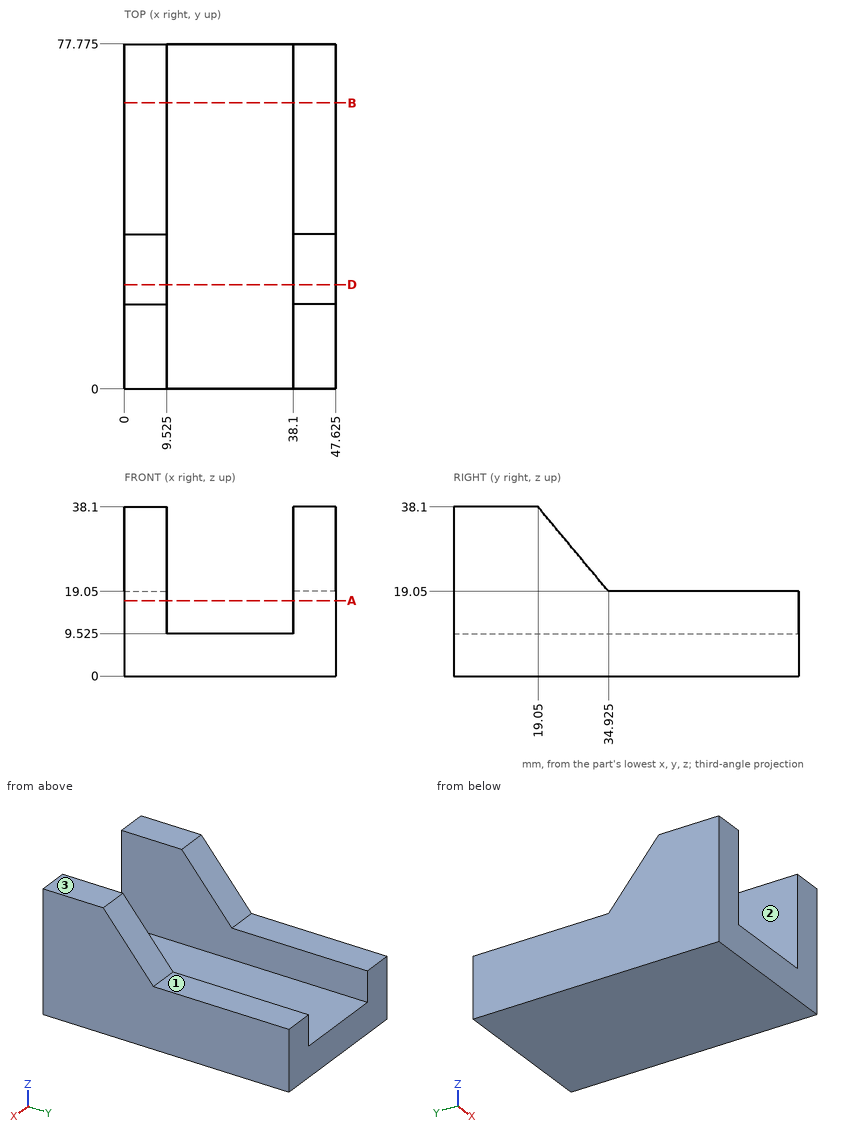
Geometry check sheet. Reference: drawing and pictorial views, mm from the part's lowest x, y, z. A direction names the side the tool comes from. Round coordinates to 2 decimals unless told otherwise and drop trailing zeros. Order: outer loops, then holes, each group sorted by start corner. A loop starts at its lowest first (then second) coordinate and runs counter-clockwise, first axis right, second up.
Q1. Depth check by flat-ended pin: P1, Ø10.5, axis at x = 44.5, y = 51, coming from the +Z side; P2, Ø8.5, axis at x = 18, y = 49, coming from the +Z side (3 decimals). Enter the tip coordinate at first touch or a pass-through.
Filled sheet:
P1: stops at z = 19.05
P2: stops at z = 9.525
Q2. Set-up check for the marked faces 1, 2 and 3: record each of +Z, -Z, +X, -X, +Y, -Y from which the full face is reachable in a straight line by a thin tool's end or side.
Filled sheet:
face 1: +Z, +X, -X, +Y
face 2: +Z, +Y, -Y
face 3: +Z, +X, -X, +Y, -Y
Q3. Cross-section at A-A, the plane z = 17. Enter the section's corners in (x, y) (1 decimal).
Filled sheet:
outline: (0, 0) - (9.5, 0) - (9.5, 77.8) - (0, 77.8) - close; (38.1, 0) - (47.6, 0) - (47.6, 77.8) - (38.1, 77.8) - close
Q4. Cross-section at B-B, the plane y = 64.5. Enter the section's corners in (x, z) (3 decimals).
Filled sheet:
outline: (0, 0) - (47.625, 0) - (47.625, 19.05) - (38.1, 19.05) - (38.1, 9.525) - (9.525, 9.525) - (9.525, 19.05) - (0, 19.05) - close
Q5. Cross-section at D-D, the plane y = 23.5. Enter the section's corners in (x, z) (3 decimals), plus the area to 3 significant figures.
Filled sheet:
outline: (0, 0) - (47.625, 0) - (47.625, 32.76) - (38.1, 32.76) - (38.1, 9.525) - (9.525, 9.525) - (9.525, 32.76) - (0, 32.76) - close
area: 896 mm2
Q6. Scan lines: L1, parallel to X at y = 62, z = 17 (3 decimals); L2, parallel to Z at x = 13.5, y = 73 (3 decimals); L3, parallel to Z at x = 41, y = 40. Record each from-to range of solid material in increasing order.
Filled sheet:
L1: x = 0 to 9.525, 38.1 to 47.625
L2: z = 0 to 9.525
L3: z = 0 to 19.05
